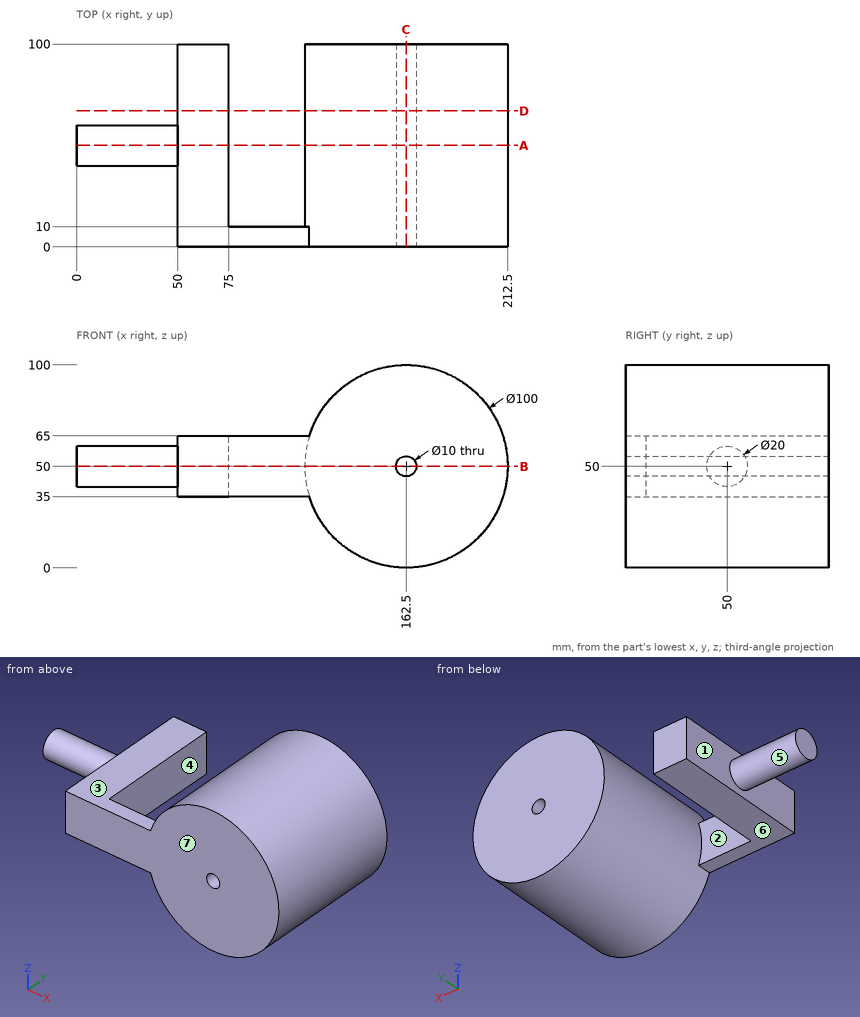
Print and shaded views of the part. All mm, measured from the part's lowest x, y and z. A direction names the side the tool comes from. Coordinates: 2 decimals unless noted, no trailing zeros. Loops run counter-clockwise (first coordinate to the right, second up) from the corner with the lowest first, then second, coordinate; pieces in that order, holes last. Notation, with made-up numbers: (25, -8.75) - (47, -8.75) arc R5 cw to (47, -2.75) - close; hole circle Ø8 at (-39, 4.25). An arc over 180 degrees is marked (long way). Use one line per item in the form item = value. Start each with the question number.
1) Flat gauge pins, fed straight in: pin 1 (4 mm diameter, centred on x = 124.5, z = 60, fed in from -Y); pin 2 (4 mm diameter, centred on x = 72.5, y = 51.5, fed in from +Z); pin 3 (3 mm diameter, centred on y = 25, z = 24, fed in from +X); pin 4 (1.5 mm diameter, centred on y = 32, z = 50, fed in from -X). Where does each tip first touch, or does it go through?
2) Drill centre lines: L1, parallel to X at y = 39, z = 50; L2, parallel to X at y = 59, z = 50; L3, parallel to Z at x = 162, y = 31. Where is each one in solid material? Low to high. Write a range as from..to.
3) Band-saw the part on C-C (x = 162.5). Give the cut face in (y, z).
4) Band-saw the part on D-D (y = 67). Give the cut face in (x, z), and give its area (3 significant figures).
5) Band-saw the part on B-B (z = 50). Give the cut face in (x, y).
6) Tool access for the marked faces 5, 6 and 7: list every direction of +Z, -Z, +X, -X, +Y, -Y with a clear straight run to the whole face (end or side of a thin tool).
7) Band-saw the part on A-A (y = 50). Give the cut face in (x, z).
8) Two-plate mould, pull along X, no slides. Class the marked faces 1, 2, 3 and 4: +X half, -X half, draft (parallel to the pull), parting line (faces both ways), or undercut.
Check values:
q1.pin_1 = 0
q1.pin_2 = 65
q1.pin_3 = 206.09
q1.pin_4 = 50
q2.L1 = 50..75, 112.5..157.5, 167.5..212.5
q2.L2 = 0..75, 112.5..157.5, 167.5..212.5
q2.L3 = 0..45.03, 54.97..100
q3.outline = (0, 0) - (100, 0) - (100, 45) - (0, 45) - close; (0, 55) - (100, 55) - (100, 100) - (0, 100) - close
q4.outline = (50, 35) - (75, 35) - (75, 65) - (50, 65) - close; circle Ø100 at (162.5, 50); hole circle Ø10 at (162.5, 50)
q4.area = 8,530 mm2
q5.outline = (0, 40) - (50, 40) - (50, 0) - (157.5, 0) - (157.5, 100) - (112.5, 100) - (112.5, 10) - (75, 10) - (75, 100) - (50, 100) - (50, 60) - (0, 60) - close; (167.5, 0) - (212.5, 0) - (212.5, 100) - (167.5, 100) - close
q6.face_5 = -X
q6.face_6 = -Z, -X, +Y, -Y
q6.face_7 = +Z, -Z, +X, -X, -Y
q7.outline = (0, 40) - (50, 40) - (50, 35) - (75, 35) - (75, 65) - (50, 65) - (50, 60) - (0, 60) - close; circle Ø100 at (162.5, 50); hole circle Ø10 at (162.5, 50)
q8.face_1 = -X half
q8.face_2 = undercut
q8.face_3 = draft
q8.face_4 = undercut
